from build123d import *

# Parameters (mm, degrees)
SKETCH1_W                        = 35.56
SKETCH1_H                        = 91.44
EXTRUDE1_DEPTH                   = 2.54
F_28_0_1405_DIAMETER_HOLE1_D     = 3.5687
F_28_0_1405_DIAMETER_HOLE1_DEPTH = 15.24
F_28_0_1405_DIAMETER_HOLE1_TIP   = 1.072145646
EXTRUDE2_DEPTH                   = 10.16
SKETCH7_W                        = 7.62
SKETCH7_H                        = 30.48
EXTRUDE3_DEPTH                   = 10.16


with BuildPart() as part:
    # Sketch1 → Extrude1 (new body)
    with BuildSketch(Plane.XY):
        Rectangle(SKETCH1_W, SKETCH1_H)
    extrude(amount=EXTRUDE1_DEPTH)

    # Sketch3 → 1/8 (0.125) Diameter Hole1 (revolve, cut)
    with BuildSketch(Plane(origin=(14.478, 41.91, 2.54), x_dir=(0, -1, 0), z_dir=(1, 0, 0))):
        Polygon((0, 0), (0, 16.193866233), (1.5875, 15.24), (1.5875, 0), align=None)
    f_1_8_0_125_diameter_hole1 = revolve(axis=Axis((14.478, 41.91, 8.89), (0, 0, -1)), mode=Mode.SUBTRACT)

    # Mirror1: 1/8 (0.125) Diameter Hole1 across plane
    add(f_1_8_0_125_diameter_hole1.mirror(Plane(origin=(0, 0, 0), x_dir=(0, 0, 1), z_dir=(1, 0, 0))), mode=Mode.SUBTRACT)

    # Mirror2: 1/8 (0.125) Diameter Hole1 across plane
    add(f_1_8_0_125_diameter_hole1.mirror(Plane.ZX), mode=Mode.SUBTRACT)

    # Mirror2 copy 1 sketch → Mirror2 copy 1 (revolve, cut)
    with BuildSketch(Plane(origin=(-14.478, -41.91, 2.54), x_dir=(0, 1, 0), z_dir=(-1, 0, 0))):
        Polygon((0, 0), (0, 16.193866233), (1.5875, 15.24), (1.5875, 0), align=None)
    revolve(axis=Axis((-14.478, -41.91, 8.89), (0, 0, -1)), mode=Mode.SUBTRACT)

    # #28 (0.1405) Diameter Hole1
    with Locations(Plane(origin=(0, -34.29, 2.54), x_dir=(1, 0, 0), z_dir=(0, 0, 1))):
        with Locations((0, 0), (0, 74.639874629)):
            Hole(F_28_0_1405_DIAMETER_HOLE1_D / 2, depth=F_28_0_1405_DIAMETER_HOLE1_DEPTH)
            with Locations((0, 0, -(F_28_0_1405_DIAMETER_HOLE1_DEPTH + F_28_0_1405_DIAMETER_HOLE1_TIP / 2))):  # 118° drill point
                Cone(0, F_28_0_1405_DIAMETER_HOLE1_D / 2, F_28_0_1405_DIAMETER_HOLE1_TIP, mode=Mode.SUBTRACT)

    # Sketch6 → Extrude2 (add)
    with BuildSketch(Plane.XY.offset(2.54)):
        Polygon((0, -45.72), (10.16, -45.72), (10.16, -38.1), (-10.16, -38.1), (-10.16, -45.72), align=None)
    extrude(amount=EXTRUDE2_DEPTH)

    # Sketch7 → Extrude3 (add)
    with BuildSketch(Plane.XY.offset(2.54)):
        with Locations((13.97, 20.32)):
            Rectangle(SKETCH7_W, SKETCH7_H)
    extrude(amount=EXTRUDE3_DEPTH)


solid = part.part
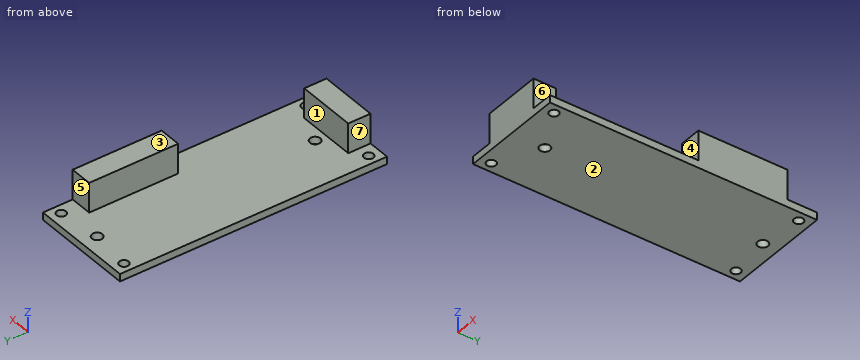
Work out the finished part from the listing and answer in its coordinate system (mm). Face numbers are marked on the shaded views. A direction names the side the tool comes from. Give positions to 0.01 mm unless a question says otherwise; leave off trailing zeros. Order: outer loops, then holes, each group sorted by start corner. A loop starts at its lowest first (then second) coordinate and runs counter-clockwise, first axis right, second up. Notation, with made-up numbers: (-14, 88.5) -> (40, 88.5) arc R26 cw to (40, 105.5) -> close; hole circle Ø2 at (40, -4.5). An arc over 180 degrees is marked (long way). One line per item, written item: value.
Item 1: Determine the mould class of the marked faces 1, 2 and 3 for opening direction Z: released by +Z, released by -Z, zero draft, split by the parting line, or undercut.
Answer sheet:
face 1: zero draft
face 2: released by -Z
face 3: released by +Z
Item 2: Find section A-A, the plane y = -41.91. Give the vertices of the cut face in (x, z).
Answer sheet:
outline: (-17.78, 0) -> (-16.07, 0) -> (-16.07, 2.54) -> (-17.78, 2.54) -> close; (-12.89, 0) -> (12.89, 0) -> (12.89, 2.54) -> (10.16, 2.54) -> (10.16, 12.7) -> (-10.16, 12.7) -> (-10.16, 2.54) -> (-12.89, 2.54) -> close; (16.07, 0) -> (17.78, 0) -> (17.78, 2.54) -> (16.07, 2.54) -> close
Item 3: A tool of negligible diameter and unlimited length cuts with its end or side. For the marked faces 4, 5, 6 and 7, from which of +Z, -Z, +X, -X, +Y, -Y can it reach the whole face along a straight path? Write none if from no direction.
Answer sheet:
face 4: +Z, +X, -X, -Y
face 5: +Z, +X, -X, +Y
face 6: +Z, +X, -Y
face 7: +Z, -X, +Y, -Y
Item 4: Find section D-D, the plane x = -8.5. Give the vertices of the cut face in (y, z).
Answer sheet:
outline: (-45.72, 0) -> (45.72, 0) -> (45.72, 2.54) -> (-38.1, 2.54) -> (-38.1, 12.7) -> (-45.72, 12.7) -> close
Item 5: Straight lines are drawn through the part: probe 1 along X at (y, z) = (-41.91, 0.8); probe 2 along Y at (x, z) = (0, 1.6); probe 3 along X at (y, z) = (41.91, 0.9). For each, find the intervals that lie inside material, in ascending order.
Answer sheet:
probe 1: -17.78 to -16.07, -12.89 to 12.89, 16.07 to 17.78
probe 2: -45.72 to -36.07, -32.51 to 38.57, 42.13 to 45.72
probe 3: -17.78 to -16.07, -12.89 to -0.87, 0.87 to 12.89, 16.07 to 17.78
Item 6: Flat-ended cylindrical pins translate along their axes: P1, Ø6, axis at x = 1, y = 15, coming from the +Z side; P2, Ø2.5, axis at y = -40.5, z = 9, coming from the +X side; P3, Ø2, axis at y = 8.5, z = 6, coming from the -X side. Find the tip coordinate at first contact, or state that the pin passes through.
Answer sheet:
P1: z = 2.54
P2: x = 10.16
P3: x = 10.16
Item 7: Find section C-C, the plane x = 0. Give the vertices of the cut face in (y, z), plus the area to 3 significant figures.
Answer sheet:
outline: (-45.72, 0) -> (-36.07, 0) -> (-36.07, 2.54) -> (-38.1, 2.54) -> (-38.1, 12.7) -> (-45.72, 12.7) -> close; (-32.51, 0) -> (38.57, 0) -> (38.57, 2.54) -> (-32.51, 2.54) -> close; (42.13, 0) -> (45.72, 0) -> (45.72, 2.54) -> (42.13, 2.54) -> close
area: 292 mm²
Item 8: Find section B-B, the plane z = 5.75. Give the vertices of the cut face in (x, y), plus the area to 3 significant figures.
Answer sheet:
outline: (-10.16, -45.72) -> (10.16, -45.72) -> (10.16, -38.1) -> (-10.16, -38.1) -> close; (10.16, 5.08) -> (17.78, 5.08) -> (17.78, 35.56) -> (10.16, 35.56) -> close
area: 387 mm²
